from build123d import *

# Parameters (mm, degrees)
SKETCH_2_R          = 1.6
CUT_EXTRUDE_1_DEPTH = 10


with BuildPart() as part:
    # Sketch 1 → Revolve 5 (revolve)
    with BuildSketch(Plane.XY):
        with BuildLine():
            Line((-11.5, 0.961485209), (-22.420203846, 0.961485209))
            Line((-22.420203846, 0.961485209), (-22.420203846, -1.538514791))
            Line((-22.420203846, -1.538514791), (-12.404957567, -1.538514791))
            ThreePointArc((-12.404957567, -1.538514791), (-8.277033439, -9.367001518), (0, -12.5))
            Line((0, -12.5), (0, 0.961485209))
            Line((0, 0.961485209), (-8.348478365, 0.961485209))
            Line((-8.348478365, 0.961485209), (-8.760960883, 0.961485209))
            ThreePointArc((-8.760960883, 0.961485209), (-8.455804212, 1.983114098), (-8.031969161, 2.961485209))
            Line((-8.031969161, 2.961485209), (-9.978754751, 2.961485209))
            Line((-9.978754751, 2.961485209), (-11.5, 0.961485209))
        make_face()
    revolve(axis=Axis((0, 0, 0), (0, 1, 0)))

    # Sketch 1_6 → Revolve 8 (revolve)
    with BuildSketch(Plane.XY):
        with BuildLine():
            Line((0, 7.5), (0, 0.961485209))
            Line((0, 0.961485209), (8.348478365, 0.961485209))
            ThreePointArc((8.348478365, 0.961485209), (5.302104928, 5.670819301), (0, 7.5))
        make_face()
    revolve(axis=Axis((0, 0, 0), (0, 1, 0)))

    # Sketch 2 → Cut-Extrude 1 (cut)
    with BuildSketch(Plane(origin=(0, 0.961485209, 0), x_dir=(1, 0, 0), z_dir=(0, 1, 0))):
        with Locations(Location((-15.5, 0, 0), (0, 0, 180))):
            Circle(SKETCH_2_R)
        with Locations(Location((15.5, 0, 0), (0, 0, 180))):
            Circle(SKETCH_2_R)
    extrude(amount=-CUT_EXTRUDE_1_DEPTH, mode=Mode.SUBTRACT)


solid = part.part
The listing builds one solid part. Answer for the finished solid, in the listing's coordinates (mm). A direction names the side the tool comes from. Give positions to 0.01 mm unless a question says otherwise; leave off trailing zeros. Write each loop counter-clockwise with the first axis right and the second up, starting at its lowest first coordinate (ties: lowest second). Pieces come first, ordered by that corner, then holes.
Item 1: Which of the six approach directions +Z, -Z, +X, -X, +Y, -Y give full straight-line access (tool end or side, diameter ignored) to faces 5 (the cylindrical face through (2.92, -0.31, 22.23)), 6 (the flat face through (10, 0.961, -10)), 7 (the flat face through (8, 0.961, -3))?
Item 2: Flat-ended cylindrical pins translate along their axes: P1, Ø1.5, axis at x = 10, y = 4, coming from the -Z side (3 decimals); P2, Ø4, axis at x = 15.5, z = 0, coming from the +Y side; P3, Ø1, axis at y = -1, z = -14, coming from the -X side; P4, Ø8, axis at x = 0.5, y = -2.5, coming from the +Z side. Find the tip coordinate at first contact, or state that the pin passes through.
Item 3: Section B-B, the plane y = 2 is taken. Write down the section's boundary in (x, z).
Item 4: Section D-D, the plane x = 0 is taken. Write down the section's boundary in (y, z).
Item 5: Section C-C, the plane x = -15.5 is taken. Write down the section's boundary in (y, z).
Item 6: Section A-A, the plane z = 0 is taken. Write down the section's boundary in (x, y).
Item 7: Determine the mould class of faces 1 (the cylindrical face through (17.1, -0.27, 0.07)), 2 (the flat face through (-10, -1.539, -10)), 3 (the cylindrical face through (-13.9, -0.27, 0.07)), 4 (the conical face through (2.18, 2.84, -9.83)) for opening direction Z: released by +Z, released by -Z, zero draft, split by the parting line, or undercut.
Item 8: Find the intervals of material crossed by line 1 along X through (y, z) = (2, 5.5); line 2 along Z through (x, y) = (2, 1) (3 decimals); line 3 along X through (y, z) = (0, -14.5), in increasing order.
Completed:
1. face 5: +Y, -Y
1. face 6: +Y
1. face 7: none
2. P1: passes through
2. P2: stops at y = 0.96
2. P3: stops at x = -17.9
2. P4: stops at z = 22.42
3. outline: circle Ø21.42 at (0, 0); circle Ø16.04 at (0, 0); hole circle Ø16.9 at (0, 0)
4. outline: (-1.54, -22.42) - (0.96, -22.42) - (0.96, -11.5) - (2.96, -9.98) - (2.96, -8.03) arc R9 cw to (0.96, -8.76) - (0.96, -8.35) arc R8.6 ccw to (0.96, 8.35) - (0.96, 8.76) arc R9 cw to (2.96, 8.03) - (2.96, 9.98) - (0.96, 11.5) - (0.96, 22.42) - (-1.54, 22.42) - (-1.54, 12.4) arc R12.5 ccw to (-1.54, -12.4) - close
5. outline: (-1.54, -16.2) - (0.96, -16.2) - (0.96, -1.6) - (-1.54, -1.6) - close; (-1.54, 1.6) - (0.96, 1.6) - (0.96, 16.2) - (-1.54, 16.2) - close
6. outline: (-22.42, -1.54) - (-17.1, -1.54) - (-17.1, 0.96) - (-22.42, 0.96) - close; (-13.9, -1.54) - (-12.4, -1.54) arc R12.5 ccw to (12.4, -1.54) - (13.9, -1.54) - (13.9, 0.96) - (11.5, 0.96) - (9.98, 2.96) - (8.03, 2.96) arc R9 cw to (8.76, 0.96) - (8.35, 0.96) arc R8.6 ccw to (-8.35, 0.96) - (-8.76, 0.96) arc R9 cw to (-8.03, 2.96) - (-9.98, 2.96) - (-11.5, 0.96) - (-13.9, 0.96) - close; (17.1, -1.54) - (22.42, -1.54) - (22.42, 0.96) - (17.1, 0.96) - close
7. face 1: undercut
7. face 2: zero draft
7. face 3: undercut
7. face 4: split by the parting line
8. line 1: x = -9.19 to -6.41, -5.84 to 5.84, 6.41 to 9.19
8. line 2: z = -11.295 to -8.52, -8.095 to 8.095, 8.52 to 11.295
8. line 3: x = -17.1 to 17.1
